Check sheet for the modelled part. Datum: model origin and axes. Units: mm. A direction names the side the tool comes from. Give positions to 0.01 mm unless a question says otherwise; leave off trailing zeros. Write each loop counter-clockwise with the first axis right and the second up, starting at its lowest first coordinate (ties: lowest second). Pieces come first, ordered by that corner, then holes.
from build123d import *

# Parameters (mm, degrees)
CROQUIS1_R              = 11.25
SALIENTE_EXTRUIR1_DEPTH = 35.8
CHAFL_N1_SIZE           = 1.5
CROQUIS3_W              = 1.5
CROQUIS3_H              = 0.8
SALIENTE_EXTRUIR2_DEPTH = 7


with BuildPart() as part:
    # Croquis1 → Saliente-Extruir1 (new body)
    with BuildSketch(Plane(origin=(0, 0, 0), x_dir=(1, 0, 0), z_dir=(0, 1, 0))):
        with Locations(Location((0, 0, 0), (0, 0, 90))):
            Circle(CROQUIS1_R)
    extrude(amount=SALIENTE_EXTRUIR1_DEPTH)

    # Chaflán1
    chafl_n1_edges = [part.edges().sort_by_distance(p)[0] for p in [
        (0, 0, 11.25),
        (0, 35.8, 11.25),
    ]]
    chamfer(chafl_n1_edges, length=CHAFL_N1_SIZE)

    # Croquis3 → Saliente-Extruir2 (add)
    with BuildSketch(Plane.XZ):
        with Locations((-4.5, 3)):
            Rectangle(CROQUIS3_W, CROQUIS3_H)
        with Locations((4.5, -3)):
            Rectangle(CROQUIS3_W, CROQUIS3_H)
    extrude(amount=SALIENTE_EXTRUIR2_DEPTH)


solid = part.part
1) Sectioned sample at B-B on x = 0. Record the boundary of the cut face in (y, z).
2) Sectioned sample at C-C on y = 29.5. Record the boundary of the cut face in (x, z), then the cut area to 3 significant figures.
3) Gauge pin test, flat ends, axial feed: pin 1 (2 mm diameter, centred on y = 5, z = -2, fed in from +X); pin 2 (1.5 mm diameter, centred on x = -5, y = 25, fed in from -Z); pin 3 (4 mm diameter, centred on x = -5.5, y = 23, fed in from +Z). Record the tip position at first contact, or that the pin passes through.
4) Access from +Z, -Z, +X, -X, +Y, -Y to the whole of each face (thin tool, end or side, straight path). Record for faces 1 (the flat face through (4, -3, -3.4)), 2 (the flat face through (0, 35.8, 0)), 3 (the flat face through (4, -3, -2.6)).
5) Sectioned sample at A-A on z = 0. Record the boundary of the cut face in (x, y), then the cut area to 3 significant figures.
6) Scan lines: L1, parallel to Y at x = 6.25, z = 2.75; L2, parallel to Z at x = -7.25, y = 14.5; L3, parallel to X at y = 29, z = 7.5. Record each from-to range of solid material in increasing order.
Answers below:
1. outline: (0, -9.75) - (1.5, -11.25) - (34.3, -11.25) - (35.8, -9.75) - (35.8, 9.75) - (34.3, 11.25) - (1.5, 11.25) - (0, 9.75) - close
2. outline: circle Ø22.5 at (0, 0)
2. area: 398 mm2
3. pin 1: stops at x = 11.21
3. pin 2: stops at z = -10.42
3. pin 3: stops at z = 10.69
4. face 1: -Z, +X, -X, -Y
4. face 2: +Z, -Z, +X, -X, +Y
4. face 3: +Z, +X, -X, -Y
5. outline: (-11.25, 1.5) - (-9.75, 0) - (9.75, 0) - (11.25, 1.5) - (11.25, 34.3) - (9.75, 35.8) - (-9.75, 35.8) - (-11.25, 34.3) - close
5. area: 801 mm2
6. L1: y = 0 to 35.8
6. L2: z = -8.6 to 8.6
6. L3: x = -8.39 to 8.39
